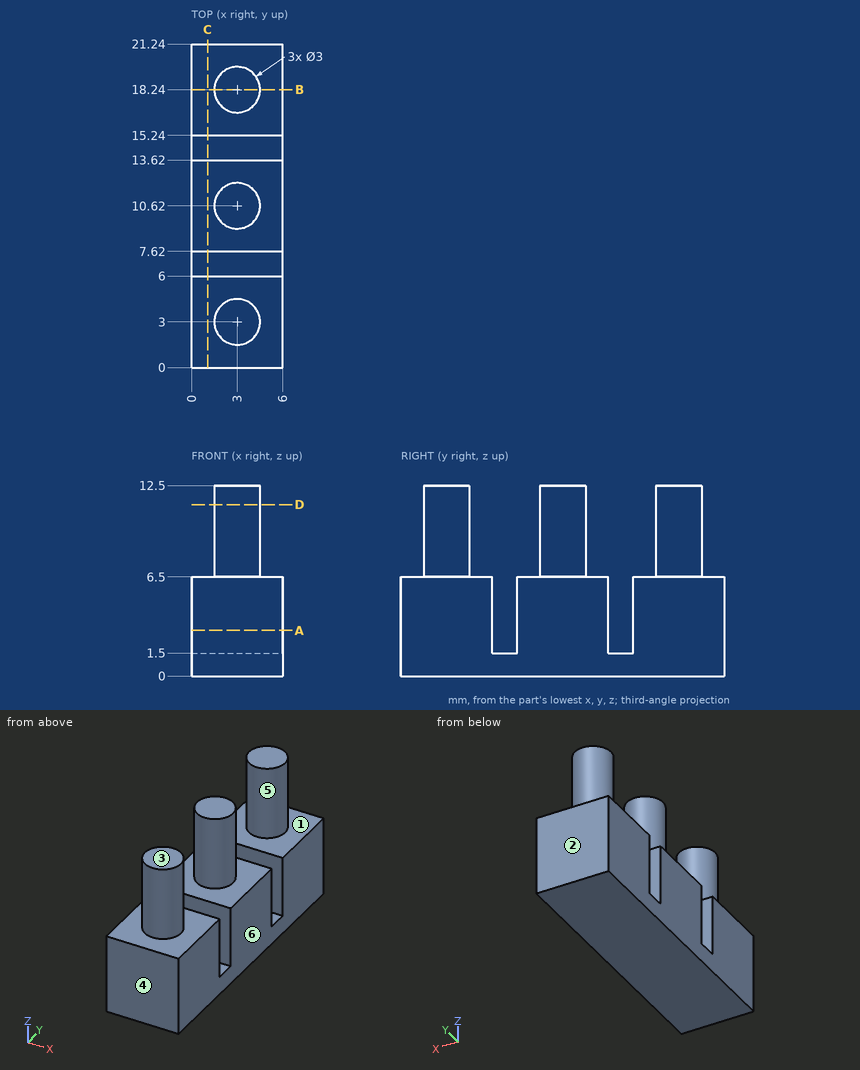
Design review of the part shown in the three views and the two pictorial views. Dimensions are in mm from the part's minimum x, y and z. A direction names the side the tool comes from. Round coordinates to 2 decimals unless told otherwise and drop trailing zeros. Write each loop counter-clockwise with the first axis right and the second up, starting at its lowest first coordinate (ties: lowest second). Pieces come first, ordered by that corner, then holes. Notation, with made-up numbers: (-16.75, 2) - (6.25, 2) arc R12 ccw to (6.25, 22) - close; hole circle Ø2 at (32.5, 31). An arc over 180 degrees is marked (long way). Write item = value, one per line. Start each with the question number.
1. Draft analysis for pull direction Y (two halves, no side actions). For the marked faces 1, 2, 3 and 4, state which applies: released by +Y, released by -Y, zero draft, split by the parting line, or undercut.
2. Wall thickness on L1, parallel to Y at x = 5.65, z = 4.5; L2, parallel to Y at x = 3.05, z = 10.75; L3, parallel to Z at x = 2, y = 5.75: over which ranges is each line inside the solid? List them lowest first.
3. Consider section B-B on y = 18.24. State the section outline as (x, z) points, plus the area to 3 significant figures.
4. Consider section D-D on z = 11.25. State the section outline as (x, y) points, plus the area to 3 significant figures.
5. Consider section C-C on x = 1.05. State the section outline as (y, z) points, plus the area to 3 significant figures.
6. For pin 1 Ø4 at (y, z) = (16, 9.5) entering from -X; pin 2 Ø1 at (x, z) = (4.5, 9) entering from +Y; pin 3 Ø1.3 at (x, y) = (3, 14.5) entering from +Z, all flat-tipped, find the tip position at first contact; note any pin that passes through.
7. For the marked faces 5 and 6, list the 3-axis set-ups (+Z, -Z, +X, -X, +Y, -Y) from which the entire face can be reached by the end or side of a thin tool; tool diameter is ignored.
8. Consider section A-A on z = 3. State the section outline as (x, y) points, plus the area to 3 significant figures.
Evaluation:
q1.face_1 = undercut
q1.face_2 = released by +Y
q1.face_3 = zero draft
q1.face_4 = released by -Y
q2.L1 = 0 to 6, 7.62 to 13.62, 15.24 to 21.24
q2.L2 = 1.5 to 4.5, 9.12 to 12.12, 16.74 to 19.74
q2.L3 = 0 to 6.5
q3.outline = (0, 0) - (6, 0) - (6, 6.5) - (4.5, 6.5) - (4.5, 12.5) - (1.5, 12.5) - (1.5, 6.5) - (0, 6.5) - close
q3.area = 57.0 mm2
q4.outline = circle Ø3 at (3, 3); circle Ø3 at (3, 10.62); circle Ø3 at (3, 18.24)
q4.area = 21.2 mm2
q5.outline = (0, 0) - (21.24, 0) - (21.24, 6.5) - (15.24, 6.5) - (15.24, 1.5) - (13.62, 1.5) - (13.62, 6.5) - (7.62, 6.5) - (7.62, 1.5) - (6, 1.5) - (6, 6.5) - (0, 6.5) - close
q5.area = 122 mm2
q6.pin_1 = 1.52
q6.pin_2 = 19.36
q6.pin_3 = 1.5
q7.face_5 = +Z
q7.face_6 = +Z, -Z, +X, +Y, -Y
q8.outline = (0, 0) - (6, 0) - (6, 6) - (0, 6) - close; (0, 7.62) - (6, 7.62) - (6, 13.62) - (0, 13.62) - close; (0, 15.24) - (6, 15.24) - (6, 21.24) - (0, 21.24) - close
q8.area = 108 mm2
